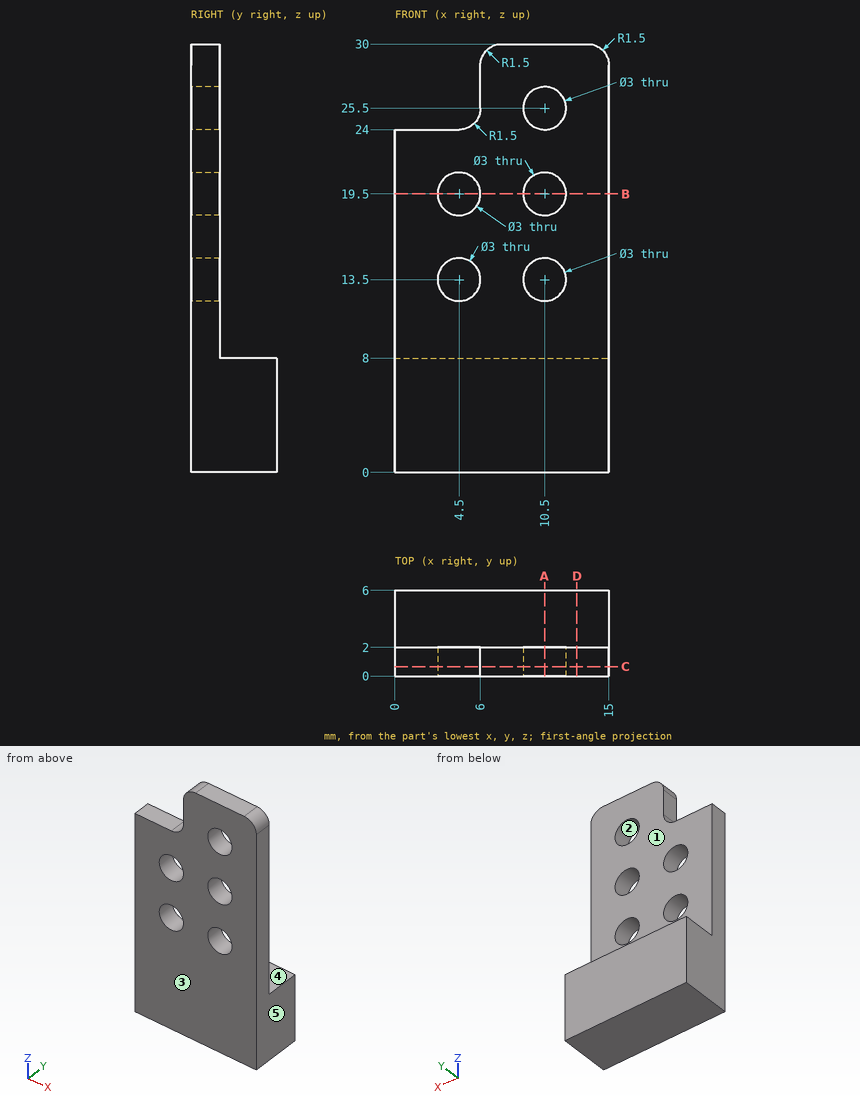
Part print with two shaded views. Sizes in mm from the minimum x, y, z corner. A direction names the side the tool comes from. Coordinates: 2 decimals unless noted, no trailing zeros. Write each loop counter-clockwise with the first axis right and the second up, starting at its lowest first coordinate (ties: lowest second). Pieces come first, ordered by that corner, then holes.
(1) Cut at A-A on x = 10.5. List the corners of the cut face in (y, z).
(2) Mould opens along Y. For the marked faces 1, 2 and 3 say: pulls with the +Y half, pulls with the -Y half, needs draft (parallel to the pull), parting line crosses it, or undercut.
(3) Drill centre lines: line 1 (Z direction, x = 10.5, y = 1.5); line 2 (Z direction, x = 4.5, y = 1.3); line 3 (Z direction, x = 13.75, y = 3.4). Where is each one in solid material? Low to high.
(4) Pin check, flat tips, straight feed: pin 1 Ø2 at (y, z) = (1, 26.5) entering from -X; pin 2 Ø0.6 at (x, y) = (1.5, 0.5) entering from +Z; pin 3 Ø4 at (x, z) = (4.5, 13.5) entering from +Y. Stop position of each tip, or through.
(5) Cut at B-B on z = 19.5. List the corners of the cut face in (x, y), and give its area (3 significant figures).
(6) Cut at D-D on x = 12.75. List the corners of the cut face in (y, z).
(7) 3-axis set-ups, long thin cutter, end or side, ignore diameter. For the marked faces 4 and 5: which of +Z, -Z, +X, -X, +Y, -Y reach the whole face in a straight line?
(8) Cut at C-C on y = 0.65. List the corners of the cut face in (x, z), and give its area (3 significant figures).
Working result:
1. outline: (0, 0) - (6, 0) - (6, 8) - (2, 8) - (2, 12) - (0, 12) - close; (0, 15) - (2, 15) - (2, 18) - (0, 18) - close; (0, 21) - (2, 21) - (2, 24) - (0, 24) - close; (0, 27) - (2, 27) - (2, 30) - (0, 30) - close
2. face 1: pulls with the +Y half
2. face 2: needs draft
2. face 3: pulls with the -Y half
3. line 1: z = 0 to 12, 15 to 18, 21 to 24, 27 to 30
3. line 2: z = 0 to 12, 15 to 18, 21 to 24
3. line 3: z = 0 to 8
4. pin 1: stops at x = 6
4. pin 2: stops at z = 24
4. pin 3: stops at y = 2
5. outline: (0, 0) - (3, 0) - (3, 2) - (0, 2) - close; (6, 0) - (9, 0) - (9, 2) - (6, 2) - close; (12, 0) - (15, 0) - (15, 2) - (12, 2) - close
5. area: 18.0 mm2
6. outline: (0, 0) - (6, 0) - (6, 8) - (2, 8) - (2, 30) - (0, 30) - close
7. face 4: +Z, +X, -X, +Y
7. face 5: +Z, -Z, +X, +Y, -Y
8. outline: (0, 0) - (15, 0) - (15, 28.5) arc R1.5 ccw to (13.5, 30) - (7.5, 30) arc R1.5 ccw to (6, 28.5) - (6, 25.5) arc R1.5 cw to (4.5, 24) - (0, 24) - close; hole circle Ø3 at (4.5, 13.5); hole circle Ø3 at (4.5, 19.5); hole circle Ø3 at (10.5, 13.5); hole circle Ø3 at (10.5, 19.5); hole circle Ø3 at (10.5, 25.5)
8. area: 378 mm2
